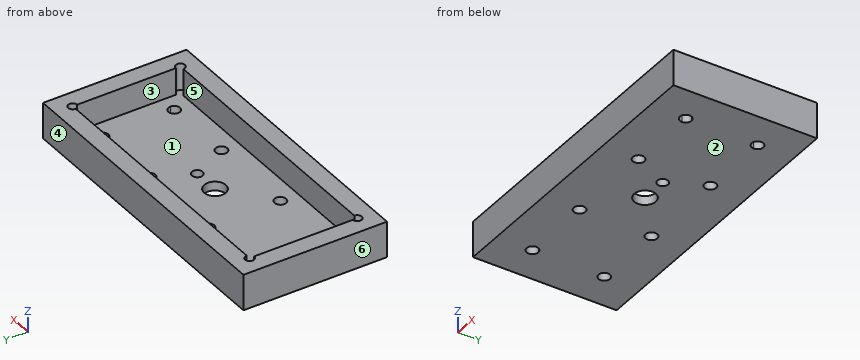
```python
from build123d import *

# Parameters (mm, degrees)
F0_W     = 170
F0_H     = 80
F1_DEPTH = 10
F2_W     = 150
F2_H     = 60
F3_DEPTH = 5
F5_DEPTH = 5
F6_R     = 6
F7_DEPTH = 5
F8_DEPTH = 10


with BuildPart() as f1:
    # F0 (on Top) → F1 (new body)
    with BuildSketch(Plane.XY):
        Rectangle(F0_W, F0_H)
    extrude(amount=F1_DEPTH)

    # F2 (on face) → F3 (cut)
    with BuildSketch(Plane.XY.offset(10)):
        Rectangle(F2_W, F2_H)
    extrude(amount=-F3_DEPTH, mode=Mode.SUBTRACT)

    # F4 (on face) → F5 (cut)
    with BuildSketch(Plane.XY.offset(10)):
        with BuildLine():
            ThreePointArc((75, 27.5), (76.767766953, 28.232233047), (77.5, 30))
            ThreePointArc((77.5, 30), (75, 32.5), (72.5, 30))
            Line((72.5, 30), (75, 30))
            Line((75, 30), (75, 27.5))
        make_face()
        with BuildLine():
            Line((75, 30), (72.5, 30))
            ThreePointArc((72.5, 30), (73.232233047, 28.232233047), (75, 27.5))
            Line((75, 27.5), (75, 30))
        make_face()
        with BuildLine():
            ThreePointArc((72.5, -30), (75, -32.5), (77.5, -30))
            ThreePointArc((77.5, -30), (76.767766953, -28.232233047), (75, -27.5))
            Line((75, -27.5), (75, -30))
            Line((75, -30), (72.5, -30))
        make_face()
        with BuildLine():
            Line((75, -30), (75, -27.5))
            ThreePointArc((75, -27.5), (73.232233047, -28.232233047), (72.5, -30))
            Line((72.5, -30), (75, -30))
        make_face()
        with BuildLine():
            Line((-75, 30), (-72.5, 30))
            ThreePointArc((-72.5, 30), (-76.767766953, 31.767766953), (-75, 27.5))
            Line((-75, 27.5), (-75, 30))
        make_face()
        with BuildLine():
            ThreePointArc((-75, 27.5), (-73.232233047, 28.232233047), (-72.5, 30))
            Line((-72.5, 30), (-75, 30))
            Line((-75, 30), (-75, 27.5))
        make_face()
        with BuildLine():
            Line((-75, -30), (-72.5, -30))
            ThreePointArc((-72.5, -30), (-73.232233047, -28.232233047), (-75, -27.5))
            Line((-75, -27.5), (-75, -30))
        make_face()
        with BuildLine():
            ThreePointArc((-75, -27.5), (-76.767766953, -31.767766953), (-72.5, -30))
            Line((-72.5, -30), (-75, -30))
            Line((-75, -30), (-75, -27.5))
        make_face()
    extrude(amount=-F5_DEPTH, mode=Mode.SUBTRACT)

    # F6 (on face) → F7 (cut)
    with BuildSketch(Plane.XY.offset(5)):
        with BuildLine():
            Line((-65, -20), (-61.75, -20))
            ThreePointArc((-61.75, -20), (-62.7019029611, -17.7019029611), (-65, -16.75))
            Line((-65, -16.75), (-65, -20))
        make_face()
        with BuildLine():
            Line((65, 20), (65, 16.75))
            ThreePointArc((65, 16.75), (67.2980970389, 17.7019029611), (68.25, 20))
            ThreePointArc((68.25, 20), (65, 23.25), (61.75, 20))
            Line((61.75, 20), (65, 20))
        make_face()
        with BuildLine():
            Line((28.25, 20), (21.75, 20))
            ThreePointArc((21.75, 20), (25, 16.75), (28.25, 20))
        make_face()
        with BuildLine():
            ThreePointArc((-21.75, -20), (-25, -16.75), (-28.25, -20))
            Line((-28.25, -20), (-21.75, -20))
        make_face()
        with BuildLine():
            ThreePointArc((-21.75, 20), (-25, 23.25), (-28.25, 20))
            Line((-28.25, 20), (-21.75, 20))
        make_face()
        with BuildLine():
            ThreePointArc((-61.75, 20), (-67.2980970389, 22.2980970389), (-65, 16.75))
            Line((-65, 16.75), (-65, 20))
            Line((-65, 20), (-61.75, 20))
        make_face()
        with BuildLine():
            ThreePointArc((-65, -16.75), (-67.2980970389, -22.2980970389), (-61.75, -20))
            Line((-61.75, -20), (-65, -20))
            Line((-65, -20), (-65, -16.75))
        make_face()
        with BuildLine():
            ThreePointArc((28.25, -20), (25, -16.75), (21.75, -20))
            Line((21.75, -20), (28.25, -20))
        make_face()
        with BuildLine():
            Line((-65, 20), (-65, 16.75))
            ThreePointArc((-65, 16.75), (-62.7019029611, 17.7019029611), (-61.75, 20))
            Line((-61.75, 20), (-65, 20))
        make_face()
        with BuildLine():
            Line((-21.75, -20), (-28.25, -20))
            ThreePointArc((-28.25, -20), (-25, -23.25), (-21.75, -20))
        make_face()
        with BuildLine():
            Line((-21.75, 20), (-28.25, 20))
            ThreePointArc((-28.25, 20), (-25, 16.75), (-21.75, 20))
        make_face()
        with BuildLine():
            Line((65, -20), (61.75, -20))
            ThreePointArc((61.75, -20), (65, -23.25), (68.25, -20))
            ThreePointArc((68.25, -20), (67.2980970389, -17.7019029611), (65, -16.75))
            Line((65, -16.75), (65, -20))
        make_face()
        with BuildLine():
            ThreePointArc((65, -16.75), (62.7019029611, -17.7019029611), (61.75, -20))
            Line((61.75, -20), (65, -20))
            Line((65, -20), (65, -16.75))
        make_face()
        with BuildLine():
            ThreePointArc((61.75, 20), (62.7019029611, 17.7019029611), (65, 16.75))
            Line((65, 16.75), (65, 20))
            Line((65, 20), (61.75, 20))
        make_face()
        with BuildLine():
            Line((28.25, -20), (21.75, -20))
            ThreePointArc((21.75, -20), (25, -23.25), (28.25, -20))
        make_face()
        with BuildLine():
            ThreePointArc((28.25, 20), (25, 23.25), (21.75, 20))
            Line((21.75, 20), (28.25, 20))
        make_face()
        Circle(F6_R)
        with BuildLine():
            ThreePointArc((18, 0), (15, 3), (12, 0))
            ThreePointArc((12, 0), (15, -3), (18, 0))
        make_face()
    extrude(amount=-F7_DEPTH, mode=Mode.SUBTRACT)

    # F8 (add): a face of the model
    f8_faces = [f1.faces().sort_by_distance(p)[0] for p in [
        (0, -38.1211705772, 10),
    ]]
    extrude(f8_faces, amount=F8_DEPTH)


solid = f1.part
```
The listing builds one solid part. Answer for the finished solid, in the listing's coordinates (mm). Face numbers are marked on the shaded views. A direction names the side the tool comes from. Give positions to 0.01 mm unless a question says otherwise; leave off trailing zeros. Order: outer loops, then holes, each group sorted by start corner. A loop starts at its lowest first (then second) coordinate and runs counter-clockwise, first axis right, second up. Notation, with made-up numbers: (87, 84.25) -> (123, 84.25) arc R15 cw to (123, 100.25) -> close; hole circle Ø3 at (51, -1). An arc over 180 degrees is marked (long way). Answer as a JSON object with one key per item and string values. Group by question number.
Item 1: A tool of negligible diameter and unlimited length cuts with its end or side. For the marked faces 1 and 2, from which of +Z, -Z, +X, -X, +Y, -Y can it reach the whole face along a straight path? Write none if from no direction.
Item 2: The part is cut by section A-A on x = 48. Write down the section's boundary in (y, z).
Item 3: Determine the mould class of the marked faces 3, 4, 5 and 6 for opening direction X: pulls with the +X half, pulls with the -X half, needs draft (parallel to the pull), parting line crosses it, or undercut.
Item 4: The part is cut by section C-C on y = 9. Write down the section's boundary in (x, z), and give its area (3 significant figures).
Item 5: Consider L1, parallel to Y at x = 25, z = 1.9; L2, parallel to X at y = -20, z = 3; L3, parallel to X at y = 23, z = 18.5. Determine where each line is inside the solid, lowest interval first. Write a range as from..to.
Item 6: The part is cut by section B-B on z = 14.75. Write down the section's boundary in (x, y).
Item 7: A flat-ended cylindrical pin translates along its axis: pin 1 (8.5 mm diameter, centred on x = 25, y = -20, fed in from +Z). Find the tip coordinate at first contact, or state that the pin passes through.
Result set:
{
 "1": {"face 1": "+Z", "face 2": "-Z, +X, -X, +Y, -Y"},
 "2": {"outline": "(-40, 0) -> (40, 0) -> (40, 20) -> (30, 20) -> (30, 5) -> (-30, 5) -> (-30, 20) -> (-40, 20) -> close"},
 "3": {"face 3": "undercut", "face 4": "needs draft", "face 5": "undercut", "face 6": "pulls with the -X half"},
 "4": {"outline": "(-85, 0) -> (85, 0) -> (85, 20) -> (75, 20) -> (75, 5) -> (-75, 5) -> (-75, 20) -> (-85, 20) -> close", "area": "1,150 mm²"},
 "5": {"L1": "-40..-23.25, -16.75..16.75, 23.25..40", "L2": "-85..-68.25, -61.75..-28.25, -21.75..21.75, 28.25..61.75, 68.25..85", "L3": "-85..-75, 75..85"},
 "6": {"outline": "(-85, -40) -> (85, -40) -> (85, 40) -> (-85, 40) -> close; hole (-75, -27.5) arc R2.5 ccw (long way) to (-72.5, -30) -> (72.5, -30) arc R2.5 ccw (long way) to (75, -27.5) -> (75, 27.5) arc R2.5 ccw (long way) to (72.5, 30) -> (-72.5, 30) arc R2.5 ccw (long way) to (-75, 27.5) -> close"},
 "7": {"pin 1": "z = 5"}
}
